Check sheet for the drawn part. Datum: minimum x, y, z corner. Units: mm. A direction names the side the tool comes from. Give positions to 0.01 mm unless a question says otherwise; leave off trailing zeros. Write each loop counter-clockwise with the first axis right and the second up, starting at its lowest first coordinate (ties: lowest second). Pieces come first, ordered by that corner, then holes. Notation, with made-up numbers: (15.25, -24) - (53.25, -24) arc R27 ccw to (53.25, 9) - close; hole circle Ø3 at (35, -15.75). An arc over 180 degrees is marked (long way). Answer as a JSON object with one key per item and string values. Group by question number.
Item 1: Tool access check on the marked faces 1 and 2. Record the directions out of +Z, -Z, +X, -X, +Y, -Y that give a thin tool (end or side, any length) a straight path to the whole face; none if there is none.
Item 2: Sectioned sample at D-D, the plane y = 35.5. Record the boundary of the cut face in (x, z), and give its area (3 significant figures).
Item 3: Sectioned sample at A-A, the plane y = 5.5. Record the boundary of the cut face in (x, z) (1 decimal), and give its area (3 significant figures).
Item 4: Sectioned sample at B-B, the plane x = 123.5. Record the boundary of the cut face in (y, z) (1 decimal), and give its area (3 significant figures).
Item 5: Sectioned sample at C-C, the plane z = 32.5. Record the boundary of the cut face in (x, y).
Item 6: Scan lines: line 1 along X through (y, z) = (2.5, 110); line 2 along X through (y, z) = (9.5, 28.5); line 3 along Z through (x, y) = (169.5, 11) (1 decimal). Record each from-to range of solid material in increasing order. Write a range as [from, to].
Item 7: Go/stop test with flat-tipped pins: pin 1 (6.5 mm diameter, centred on x = 166.5, z = 114.5, fed in from +Y); pin 2 (6.5 mm diameter, centred on x = 128, y = 30, fed in from -Z); pin 3 (6 mm diameter, centred on x = 55.5, y = 31.5, fed in from +Z). Record where each tip stops, or that it passes through.
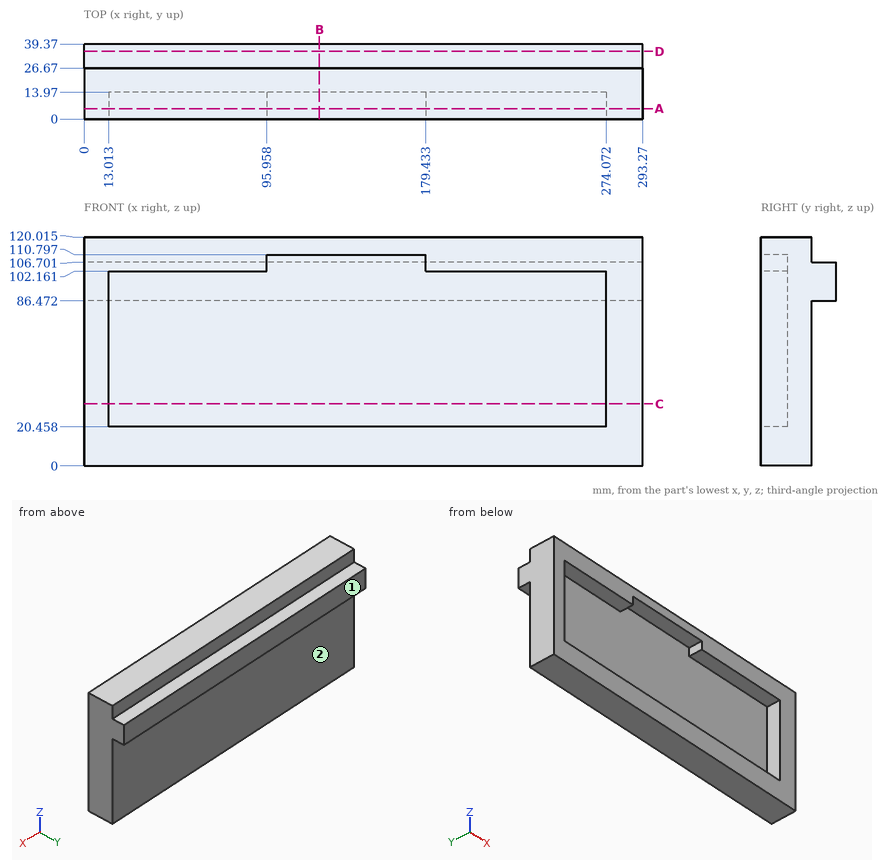
Geometry check:
{
 "1": {"face 1": "+Z, -Z, +X, -X, +Y", "face 2": "-Z, +X, -X, +Y"},
 "2": {"outline": "(0, 86.47) - (293.27, 86.47) - (293.27, 106.7) - (0, 106.7) - close", "area": "5,930 mm^2"},
 "3": {"outline": "(0, 0) - (293.3, 0) - (293.3, 120) - (0, 120) - close; hole (13, 20.5) - (274.1, 20.5) - (274.1, 102.2) - (179.4, 102.2) - (179.4, 110.8) - (96, 110.8) - (96, 102.2) - (13, 102.2) - close", "area": "13,100 mm^2"},
 "4": {"outline": "(0, 0) - (26.7, 0) - (26.7, 86.5) - (39.4, 86.5) - (39.4, 106.7) - (26.7, 106.7) - (26.7, 120) - (0, 120) - (0, 110.8) - (14, 110.8) - (14, 20.5) - (0, 20.5) - close", "area": "2,200 mm^2"},
 "5": {"outline": "(0, 0) - (13.01, 0) - (13.01, 13.97) - (274.07, 13.97) - (274.07, 0) - (293.27, 0) - (293.27, 26.67) - (0, 26.67) - close"},
 "6": {"line 1": "[0, 95.96], [179.43, 293.27]", "line 2": "[0, 13.01], [274.07, 293.27]", "line 3": "[0, 20.5], [110.8, 120]"},
 "7": {"pin 1": "y = 26.67", "pin 2": "z = 86.47", "pin 3": "z = 106.7"}
}
